from build123d import *

# Parameters (mm, degrees)
FILLET1_R          = 0.1
HEX_START          = -1.2
HEX_2_DEPTH        = 1.2
SKETCH4_R          = 5.337249995
CUT_EXTRUDE1_DEPTH = 3
CHAMFER1_SIZE      = 0.3


with BuildPart() as part:
    # BodySke → BaseBody (revolve)
    with BuildSketch(Plane.XY, mode=Mode.PRIVATE) as basebody_sk:
        Polygon((0, 0), (0, 2.85), (0.35, 2.85), (1.7, 1.5), (7.7195, 1.5), (8, 1.2195), (8, 0), align=None)
    revolve(basebody_sk.sketch.rotate(Axis((0, 0, 0), (1, 0, 0)), 90), axis=Axis((0, 0, 0), (1, 0, 0)))

    # Fillet1
    fillet1_edges = [part.edges().sort_by_distance(p)[0] for p in [
        (1.7, 0, -1.5),
    ]]
    fillet(fillet1_edges, radius=FILLET1_R)

    # Hex 2: read off the stored shape, not the designer's step
    # Hex 2 outline → Hex 2 (cut)
    with BuildSketch(Plane.ZY.offset(HEX_START)):
        Polygon((-1.01, -0.583123772), (0, -1.166247544), (1.01, -0.583123772), (1.01, 0.583123772), (0, 1.166247544), (-1.01, 0.583123772), align=None)
    extrude(amount=HEX_2_DEPTH, mode=Mode.SUBTRACT)

    # Hex 2 2 outline → Hex 2 2 (revolve, cut)
    with BuildSketch(Plane.YX):
        Polygon((1.01, 1.2), (0, 1.783123772), (0, 1.2), align=None)
    revolve(axis=Axis((0, 0, 0), (1, 0, 0)), mode=Mode.SUBTRACT)

    # Sketch4 → Cut-Extrude1 (cut)
    with BuildSketch(Plane(origin=(8, 0, 0), x_dir=(0, 0, -1), z_dir=(1, 0, 0))):
        Circle(SKETCH4_R)
    extrude(amount=-CUT_EXTRUDE1_DEPTH, mode=Mode.SUBTRACT)

    # Chamfer1
    chamfer1_edges = [part.edges().sort_by_distance(p)[0] for p in [
        (5, 0, -1.5),
    ]]
    chamfer(chamfer1_edges, length=CHAMFER1_SIZE)


solid = part.part
Read the model definition and answer for the solid it produces. Units are mm, in the model's axes. A direction names the side the tool comes from. Coordinates: 2 decimals unless noted, no trailing zeros. Order: outer loops, then holes, each group sorted by start corner. A loop starts at its lowest first (then second) coordinate and runs counter-clockwise, first axis right, second up. Notation, with made-up numbers: M 49.25,61.25 L 107.25,61.25 A24 ccw 107.25,79.25 Z; hole C 62,-39 d1. An arc over 180 degrees is marked long. Put each result on its own line as item: value. Start each with the question number.
Item 1: Consider probe 1 along Z at (x, y) = (3.35, 0.05); probe 2 along Z at (x, y) = (1.4, 0.1); probe 3 along Z at (x, y) = (0.55, 0.05). Determine where each line is inside the solid, lowest interval first. Write a range as [from, to].
Item 2: Given pin 1 Ø1.5 at (x, y) = (1.5, -2) entering from +Z, flat-ended and moving along its own axis, determine where the tip first touches the part or whether it passes through.
Item 3: The mould has two halves that part along Y. Classify faces 1 (the face through (5, 0, 0)), 2 (the face through (3.24, -0.45, 1.43)), 3 (the face through (1, 0, -1.01)): +Y half, -Y half, draft (parallel to the pull), parting line (faces both ways), or undercut.
Item 4: Section A-A, the plane x = 3.95 is taken. Determine the outline of the cut face in (y, z).
Item 5: For faces 4 (the face through (0, 0, -1.2)), 5 (the face through (0.608, 0.879, -0.498)), determine the directions among +Z, -Z, +X, -X, +Y, -Y from which every point of the face is accessible in a straight line to the end or side of a thin tool.
Computed:
1. probe 1: z = [-1.5, 1.5]
1. probe 2: z = [-1.8, -0.66], [0.66, 1.8]
1. probe 3: z = [-2.65, -1.01], [1.01, 2.65]
2. pin 1: stops at z = 1.7
3. face 1: draft
3. face 2: parting line
3. face 3: undercut
4. outline: C 0,0 d3
5. face 4: +Z, -Z, -X, +Y, -Y
5. face 5: -X
